Source: CAD feature listing. Evaluate the final solid. Frame: model axes, mm. Face numbers are marked on the shaded views. Give positions to 0.01 mm unless a question says otherwise; leave off trailing zeros. Order: outer loops, then holes, each group sorted by start corner. A loop starts at its lowest first (then second) coordinate and runs counter-clockwise, first axis right, second up. Notation, with made-up numbers: M 85.5,-1 L 97.5,-1 A9 cw 97.5,3 Z; hole C 50.25,12 d9. An arc over 180 degrees is marked long. One line per question, with ' | ' between items. Start each with the question number.
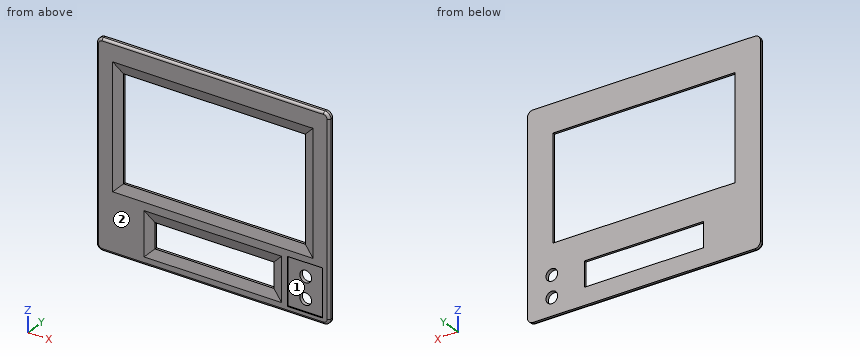
from build123d import *

# Parameters (mm, degrees)
F0_W     = 200
F0_H     = 170
F0_W_2   = 102
F0_H_2   = 21
F0_W_3   = 156
F0_H_3   = 88
F1_DEPTH = 4
F2_R     = 5
F3_R     = 5
F4_SIZE2 = 2
F4_SIZE  = 8
F5_R     = 2
F6_W     = 30
F6_H     = 40
F7_DEPTH = 1
F8_R     = 5
F9_DEPTH = 25


with BuildPart() as f1:
    # F0 (on Front) → F1 (new body)
    with BuildSketch(Plane.XZ):
        with Locations((0, 85)):
            Rectangle(F0_W, F0_H)
        with Locations((0, 25)):
            Rectangle(F0_W_2, F0_H_2, mode=Mode.SUBTRACT)
        with Locations((0, 102.15)):
            Rectangle(F0_W_3, F0_H_3, mode=Mode.SUBTRACT)
    extrude(amount=F1_DEPTH)

    # F2
    f2_edges = [f1.edges().sort_by_distance(p)[0] for p in [
        (-100, -2, 0),
    ]]
    fillet(f2_edges, radius=F2_R)

    # F3
    f3_edges = [f1.edges().sort_by_distance(p)[0] for p in [
        (100, -2, 0),
        (100, -2, 170),
        (-100, -2, 170),
    ]]
    fillet(f3_edges, radius=F3_R)

    # F4
    f4_edges = [f1.edges().sort_by_distance(p)[0] for p in [
        (-78, -4, 102.15),
        (78, -4, 102.15),
        (0, -4, 146.15),
        (0, -4, 58.15),
        (0, -4, 35.5),
        (0, -4, 14.5),
        (-51, -4, 25),
        (51, -4, 25),
    ]]
    f4_side = f1.faces().sort_by_distance((-97.375119, -4, 85))[0]
    chamfer(f4_edges, length=F4_SIZE, length2=F4_SIZE2, reference=f4_side)

    # F5
    f5_edges = [f1.edges().sort_by_distance(p)[0] for p in [
        (0, -4, 0),
    ]]
    fillet(f5_edges, radius=F5_R)

    # F6 (on face) → F7 (cut)
    with BuildSketch(Plane.XZ.offset(4)):
        with Locations((79, 25)):
            Rectangle(F6_W, F6_H)
    extrude(amount=-F7_DEPTH, mode=Mode.SUBTRACT)

    # F8 (on face) → F9 (cut)
    with BuildSketch(Plane.XZ.offset(3)):
        with Locations((79, 15)):
            Circle(F8_R)
        with Locations((79, 33)):
            Circle(F8_R)
    extrude(amount=-F9_DEPTH, mode=Mode.SUBTRACT)


solid = f1.part
Item 1: Pin query (flat end, axial travel): pin 1 Ø0.8 at (y, z) = (-3.5, 19.5) entering from +X; pin 2 Ø0.5 at (x, y) = (81, -3.5) entering from +Z; pin 3 Ø15 at (x, z) = (79.5, 27.5) entering from -Y. Return the tip coordinate at first contact, or that it passes through.
Item 2: Cut plane D-D on x = -55. Return the cut outline in (y, z), and give its area (3 significant figures).
Item 3: Cut plane B-B on y = -0.8. Return the cut outline in (x, z).
Item 4: Cut plane C-C on z = 60.5. Return the cut outline in (x, y).
Item 5: Mould query, pull axis X, two halves, no side actions, for the marked faces 1 and 2. Classes: pulls with the +X half, pulls with the -X half, needs draft (parallel to the pull), parting line crosses it, or undercut.
Item 6: Line query: line 1 (Z direction, x = 79, y = -0.9); line 2 (Z direction, x = 29, y = -0.55); line 3 (Z direction, x = 54, y = -0.35). Output: solid intervals per line, ascending.
Item 7: Cut plane A-A on x = -32. Return the cut outline in (y, z), and give its area (3 significant figures).
Results are:
1) pin 1: stops at x = 99.67 | pin 2: stops at z = 169.56 | pin 3: stops at y = -3
2) outline: M -4,2 A2 ccw -2,0 L 0,0 L 0,58.15 L -2,58.15 L -4,50.15 L -4,43.5 L -3,39.5 L -3,10.5 L -4,6.5 Z; M -4,154.15 L -2,146.15 L 0,146.15 L 0,170 L -2,170 A2 ccw -4,168 Z | area: 277 mm2
3) outline: M -100,5 A5 ccw -95,0 L 95,0 A5 ccw 100,5 L 100,165 A5 ccw 95,170 L -95,170 A5 ccw -100,165 Z; hole M -78,58.15 L 78,58.15 L 78,146.15 L -78,146.15 Z; hole M -51,14.5 L 51,14.5 L 51,35.5 L -51,35.5 Z; hole C 79,15 d10; hole C 79,33 d10
4) outline: M -100,-2 A2 ccw -98,-4 L -86,-4 L -78,-2 L -78,0 L -100,0 Z; M 78,-2 L 86,-4 L 98,-4 A2 ccw 100,-2 L 100,0 L 78,0 Z
5) face 1: undercut | face 2: needs draft
6) line 1: z = 0 to 10, 20 to 28, 38 to 170 | line 2: z = 0 to 14.5, 35.5 to 58.15, 146.15 to 170 | line 3: z = 0 to 58.15, 146.15 to 170
7) outline: M -4,2 A2 ccw -2,0 L 0,0 L 0,14.5 L -2,14.5 L -4,6.5 Z; M -4,43.5 L -2,35.5 L 0,35.5 L 0,58.15 L -2,58.15 L -4,50.15 Z; M -4,154.15 L -2,146.15 L 0,146.15 L 0,170 L -2,170 A2 ccw -4,168 Z | area: 210 mm2
